Source: CAD feature listing. Evaluate the final solid. Frame: model axes, mm. Give positions to 0.01 mm unless a question says otherwise; leave off trailing zeros. Order: outer loops, then holes, each group sorted by start corner. A loop starts at its lowest first (then second) coordinate and runs counter-clockwise, first axis right, second up. Notation, with made-up numbers: M 81.25,24 L 113.25,24 A6 cw 113.25,29 Z; hole C 21.5,30.25 d10. An arc over 180 degrees is marked long. Answer in a Markdown table with one row per item. Add a question column.
(1) Section query A-A, the plane z = 0. Return loops of the section in (x, y), plus the area to 3 significant figures.
(2) Section query B-B, the plane y = 2.5. Return loops of the section in (x, z), plus the area to 3 significant figures.
(3) Section query C-C, the plane y = -2.75. Return loops of the section in (x, z).
(4) Section query D-D, the plane z = -11. Return loops of the section in (x, y).
(5) Pin query (flat end, axial travel): P1, Ø1.8, axis at y = 1.72, z = -21, coming from the +X side; P2, Ø2, axis at x = -5, z = -1.5, coming from the -Y side; P3, Ø6, axis at x = -1, z = 2.5, coming from the +Y side; P4, Ø0.6, axis at y = 0, z = -4, coming from the +X side. Return the tip coordinate at first contact, or that it passes through.
(6) Mould query, pull axis X, two halves, no side actions, for faces 1 (the face through (0, -4, 0)), 2 (the face through (0, 0, -3)), 3 (the face through (-0.5, -1, -15)). Classes: pulls with the +X half, pulls with the -X half, needs draft (parallel to the pull), parting line crosses it, or undercut.
(7) Material intervals for line 1 along Y through (x, z) = (0.25, -15); line 2 along Y through (x, z) = (0.15, -21); line 3 along X through (y, z) = (-0.75, 4), sorted ascending.
from build123d import *

# Parameters (mm, degrees)
FILLET1_R                = 2
SKETCH5_R                = 8.5
SKETCH5_R_2              = 7
BOSS_EXTRUDE1_DEPTH      = 0.1
BOSS_EXTRUDE2_DEPTH      = 0.5
BOSS_EXTRUDE2_DEPTH_BACK = 0.5
SKETCH6_R                = 1.5


with BuildPart() as part:
    # Sketch4 → Revolve1 (revolve)
    with BuildSketch(Plane(origin=(0, 0, 0), x_dir=(0, 0, -1), z_dir=(1, 0, 0))):
        Polygon((0, 0), (-3.75, 0), (-4.25, -0.5), (-4.75, 0), (-8.5, 0), (-8.5, -4), (0, -4), align=None)
    revolve(axis=Axis((0, 1.890471386, 0), (0, -1, 0)))

    # Fillet1
    fillet1_edges = [part.edges().sort_by_distance(p)[0] for p in [
        (0, 0, -8.5),
    ]]
    fillet(fillet1_edges, radius=FILLET1_R)



with BuildPart() as body_2:
    # Sketch5 → Boss-Extrude1 (new body)
    with BuildSketch(Plane.XZ.offset(4)):
        with Locations(Location((0, 0, 0), (0, 0, 90))):
            Circle(SKETCH5_R)
        with Locations(Location((0, 0, 0), (0, 0, 270))):
            Circle(SKETCH5_R_2, mode=Mode.SUBTRACT)
    extrude(amount=BOSS_EXTRUDE1_DEPTH)


with BuildPart() as part_1:
    add(part.part)

    add(body_2.part)  # Boss-Extrude2 merges body 2
    # Sketch6 → Boss-Extrude2 (add, two sides: drawn at the far end of the back side and taken through both)
    with BuildSketch(Plane(origin=(0, 0, 0), x_dir=(0, 0, -1), z_dir=(1, 0, 0)).offset(-BOSS_EXTRUDE2_DEPTH_BACK)):
        with BuildLine():
            Line((16.303953204, 0), (0, 0))
            Line((0, 0), (0, -0.907670556))
            Line((0, -0.907670556), (7.174444166, -0.907670556))
            Line((7.174444166, -0.907670556), (8.5, -4))
            Line((8.5, -4), (17.632863069, -3.95))
            Line((17.632863069, -3.95), (22.328664529, 0.223690648))
            ThreePointArc((22.328664529, 0.223690648), (22.869458415, 2.429287044), (21, 3.718565415))
            Line((21, 3.718565415), (16.303953204, 0))
        make_face()
        with Locations((21, 1.718565415)):
            Circle(SKETCH6_R, mode=Mode.SUBTRACT)
    extrude(amount=BOSS_EXTRUDE2_DEPTH + BOSS_EXTRUDE2_DEPTH_BACK)


solid = part_1.part
Values follow:
| question | item | result |
|---|---|---|
| 1 | outline | M -8.5,-4.1 L -7,-4.1 L -7,-4 L 7,-4 L 7,-4.1 L 8.5,-4.1 L 8.5,-2 A2 ccw 6.5,0 L 4.75,0 L 4.25,-0.5 L 3.75,0 L -3.75,0 L -4.25,-0.5 L -4.75,0 L -6.5,0 A2 ccw -8.5,-2 Z |
| 1 | area | 66.1 mm² |
| 2 | outline | M -0.5,-22.84 L 0.5,-22.84 L 0.5,-22.28 L -0.5,-22.28 Z; M -0.5,-19.72 L 0.5,-19.72 L 0.5,-19.46 L -0.5,-19.46 Z |
| 2 | area | 0.819 mm² |
| 3 | outline | M -0.5,-18.98 L 0.5,-18.98 L 0.5,-8.49 A8.5 ccw long -0.5,-8.49 Z |
| 4 | outline | M -0.5,-3.99 L 0.5,-3.99 L 0.5,0 L -0.5,0 Z |
| 5 | P1 | passes through |
| 5 | P2 | stops at y = -4 |
| 5 | P3 | stops at y = 0 |
| 5 | P4 | stops at x = 6.44 |
| 6 | face 1 | undercut |
| 6 | face 2 | needs draft |
| 6 | face 3 | pulls with the -X half |
| 7 | line 1 | y = -3.96 to 0 |
| 7 | line 2 | y = -0.96 to 0.22, 3.22 to 3.72 |
| 7 | line 3 | x = -7 to 7 |
